from build123d import *

# Parameters (mm, degrees)
BOSS_EXTRUDE1_DEPTH = 25
BOSS_EXTRUDE1_DRAFT = -30
SHELL1_T            = -5
FILLET1_R           = 1
FILLET2_R           = 2.5
FILLET3_R           = 1


with BuildPart() as part:
    # Sketch1 → Boss-Extrude1 (with draft: the straight prism first)
    with BuildSketch(Plane(origin=(0, 0, 0), x_dir=(1, 0, 0), z_dir=(0, 1, 0))):
        with BuildLine():
            Line((-65, -40), (65, -40))
            ThreePointArc((65, -40), (72.071067812, -37.071067812), (75, -30))
            Line((75, -30), (75, 30))
            ThreePointArc((75, 30), (72.071067812, 37.071067812), (65, 40))
            Line((65, 40), (-65, 40))
            ThreePointArc((-65, 40), (-72.071067812, 37.071067812), (-75, 30))
            Line((-75, 30), (-75, -30))
            ThreePointArc((-75, -30), (-72.071067812, -37.071067812), (-65, -40))
        make_face()
    extrude(amount=BOSS_EXTRUDE1_DEPTH)
    # Boss-Extrude1: the draft: its side faces are tilted about the plane it starts from
    boss_extrude1_sides = [part.faces().sort_by_distance(p)[0] for p in [
        (0, 12.5, 40),
        (72.071067812, 12.5, 37.071067812),
        (75, 12.5, 0),
        (72.071067812, 12.5, -37.071067812),
        (0, 12.5, -40),
        (-72.071067812, 12.5, -37.071067812),
        (-75, 12.5, 0),
        (-72.071067812, 12.5, 37.071067812),
    ]]
    draft(boss_extrude1_sides, Plane(origin=(0, 0, 0), x_dir=(1, 0, 0), z_dir=(0, 1, 0)), BOSS_EXTRUDE1_DRAFT)

    # Shell1
    shell1_openings = [part.faces().sort_by_distance(p)[0] for p in [
        (0, 25, 0),
    ]]
    offset(amount=SHELL1_T, openings=shell1_openings, kind=Kind.INTERSECTION)

    # Fillet1
    fillet1_edges = [part.edges().sort_by_distance(p)[0] for p in [
        (70.02982636, 5, -35.02982636),
        (0, 5, -37.113248654),
        (-70.02982636, 5, -35.02982636),
        (-72.113248654, 5, 0),
        (-70.02982636, 5, 35.02982636),
        (0, 5, 37.113248654),
        (70.02982636, 5, 35.02982636),
        (72.113248654, 5, 0),
    ]]
    fillet(fillet1_edges, radius=FILLET1_R)

    # Fillet2
    fillet2_edges = [part.edges().sort_by_distance(p)[0] for p in [
        (-89.43375673, 25, 0),
        (0, 25, 54.43375673),
        (89.43375673, 25, 0),
        (0, 25, -48.660254038),
        (-83.660254038, 25, 0),
        (0, 25, 48.660254038),
        (83.660254038, 25, 0),
        (0, 25, -54.43375673),
    ]]
    fillet(fillet2_edges, radius=FILLET2_R - 0.0001)  # a hair under: the kernel refuses the full size

    # Fillet3
    fillet3_edges = [part.edges().sort_by_distance(p)[0] for p in [
        (-75, 0, 0),
        (-72.071067812, 0, -37.071067812),
        (0, 0, -40),
        (72.071067812, 0, -37.071067812),
        (75, 0, 0),
        (72.071067812, 0, 37.071067812),
        (0, 0, 40),
        (-72.071067812, 0, 37.071067812),
    ]]
    fillet(fillet3_edges, radius=FILLET3_R)


solid = part.part
Can you work these out from the model? Positions are in its coordinate system, mm. A direction names the side the tool comes from. Coordinates: 2 decimals unless noted, no trailing zeros. Order: outer loops, then holes, each group sorted by start corner. A loop starts at its lowest first (then second) coordinate and runs counter-clockwise, first axis right, second up. Notation, with made-up numbers: (86.25, -25.75) - (103.25, -25.75) arc R27 ccw to (103.25, 11.25) - close; hole circle Ø10 at (26, -6). An arc over 180 degrees is marked (long way). Answer as a JSON object with one key per item and string values. Group by question number.
Q1. Imagine slicing it at B-B (y = 14.25). Please give me the cut outline in (x, z).
Q2. Will these pins go through, and if not, where does the flat tip stop? P1, Ø5, axis at y = 16, z = 5.5, coming from the +X side; P2, Ø4, axis at x = 52.5, z = -4.5, coming from the +Y side; P3, Ø4, axis at y = 14, z = 8, coming from the +X side.
Q3. On a 3-axis mill with a long thin cutter (end or side, diameter ignored), from which of +Z, -Z, +X, -X, +Y, -Y can I reach the whole of each face in a straight line? I mean faces 5 (the face through (76.58, 10.73, -41.32)), 6 (the face through (74.004, 14.497, -38.809)). Say none if no direction works.
Q4. We'd pull the mould along X, two halves only. Please class faces 1 (the face through (-81.195, 10.73, -0.42)), 2 (the face through (77.6, 14.5, 0.4)), 3 (the face through (81.195, 10.73, 0.42)), 4 (the face through (-1, 5, -1)): +X half, -X half, draft (parallel to the pull), parting line (faces both ways), or undercut.
Q5. I need wall thicknesses on line 1 (Y direction, x = -54, z = -30.5); line 2 (Z direction, x = -63.5, y = 7); line 3 (Z direction, x = 40, y = 14.25). Which ranges of each line are inside material? Lowest first, please. Write a range as from..to.
Determined:
{
 "1": {"outline": "(-83.23, -30) arc R18.23 ccw to (-65, -48.23) - (65, -48.23) arc R18.23 ccw to (83.23, -30) - (83.23, 30) arc R18.23 ccw to (65, 48.23) - (-65, 48.23) arc R18.23 ccw to (-83.23, 30) - close; hole (-77.45, -30) arc R12.45 ccw to (-65, -42.45) - (65, -42.45) arc R12.45 ccw to (77.45, -30) - (77.45, 30) arc R12.45 ccw to (65, 42.45) - (-65, 42.45) arc R12.45 ccw to (-77.45, 30) - close"},
 "2": {"P1": "stops at x = 85.68", "P2": "stops at y = 5", "P3": "stops at x = 84.24"},
 "3": {"face 5": "-Z, +X, -Y", "face 6": "+Y"},
 "4": {"face 1": "-X half", "face 2": "undercut", "face 3": "+X half", "face 4": "undercut"},
 "5": {"line 1": "y = 0..5", "line 2": "z = -44.04..-38.27, 38.27..44.04", "line 3": "z = -48.23..-42.45, 42.45..48.23"}
}
